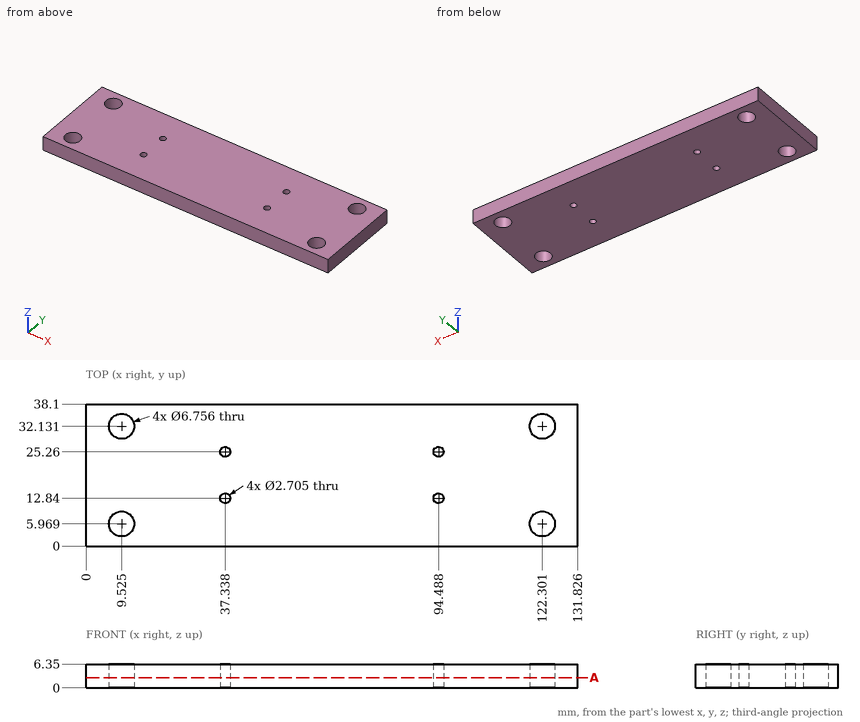
Can you work these out from the drawing? Everything is in mm from the part's minimum corner. Coordinates: 2 decimals unless noted, no trailing zeros. Put each result on its own line as item: value. Start each with the question number.
Item 1: If I drill on line 1 along X through (y, z) = (8.5, 2.5) (1 decimal); line 2 along X through (y, z) = (3.5, 1.75) (1 decimal); line 3 along Y through (x, z) = (94, 3), over which ranges is the centre line in solid material (lowest first)?
Item 2: Suppose I cut it at A-A (z = 2.75). State how many separate pieces and enclosed holes the cut face has, and give its area (3 significant figures).
Item 3: For pin 1 (2 mm diameter, centred on x = 37.34, y = 25.26, fed in from +Z); pin 2 (9 mm diameter, centred on x = 9.525, y = 32.131, fed in from +Z), each with a flat end and sliding along its axis, tell me the tip position at first contact or that it passes through.
Here are the results:
1. line 1: 0 to 7.3, 11.8 to 120.1, 124.5 to 131.8
1. line 2: 0 to 7.2, 11.8 to 120, 124.6 to 131.8
1. line 3: 0 to 11.58, 14.1 to 24, 26.52 to 38.1
2. separate pieces: 1
2. enclosed holes: 8
2. area: 4,860 mm²
3. pin 1: through
3. pin 2: z = 6.35
